Check sheet for the modelled part. Datum: model origin and axes. Units: mm. A direction names the side the tool comes from. Round coordinates to 2 decimals unless told otherwise and drop trailing zeros. Write each loop counter-clockwise with the first axis right and the second up, starting at its lowest first coordinate (ties: lowest second). Pieces come first, ordered by that corner, then holes. Notation, with made-up numbers: M 41.25,-24 L 50.25,-24 A25 cw 50.25,-4 Z; hole C 25.25,-15 d7. An arc over 180 degrees is marked long. Put each result on its own line as item: value.
```python
from build123d import *

# Parameters (mm, degrees)
F0_R     = 5
F0_R_2   = 3
F1_DEPTH = 20.162448287
F2_R     = 0.6272281394
F0_R_3   = 6
F3_DEPTH = 1.5


# Not quite as in the source:
# - a fillet or chamfer that OpenCascade refuses, or shapes differently, is made with other operations: its cross-section is extruded or revolved along the edge and cut away or added


with BuildPart() as f1:
    # F0 (on Front) → F1 (new body, symmetric)
    with BuildSketch(Plane.XZ):
        Circle(F0_R)
        Circle(F0_R_2, mode=Mode.SUBTRACT)
    extrude(amount=F1_DEPTH, both=True)

    # F2
    f2_edges = [f1.edges().sort_by_distance(p)[0] for p in [
        (-5, -20.162448, 0),
        (-5, 20.162448, 0),
    ]]
    fillet(f2_edges, radius=F2_R)

    # F0 (on Front) → F3 (join, symmetric)
    with BuildSketch(Plane.XZ):
        Circle(F0_R_3)
        Circle(F0_R, mode=Mode.SUBTRACT)
    extrude(amount=F3_DEPTH, both=True)

    # F4: fillet of radius 1.5182281224 on 2 edges, made by hand

    # F4_s1 → F4_t2 (revolve, cut)
    with BuildSketch(Plane.XY):
        with BuildLine():
            ThreePointArc((5, 1.5), (5.7251151811, 0.9442269358), (6, 0.072955416))
            Line((6, 0.072955416), (6, 1.5))
            Line((6, 1.5), (5, 1.5))
        make_face()
    revolve(axis=Axis((0, 1.5, 0), (0, -1, 0)), mode=Mode.SUBTRACT)

    # F4_s3 → F4_t4 (revolve, cut)
    with BuildSketch(Plane.XY):
        with BuildLine():
            ThreePointArc((6, -0.072955416), (5.7251151811, -0.9442269358), (5, -1.5))
            Line((5, -1.5), (6, -1.5))
            Line((6, -1.5), (6, -0.072955416))
        make_face()
    revolve(axis=Axis((0, -1.5, 0), (0, -1, 0)), mode=Mode.SUBTRACT)


solid = f1.part
```
1. Scan lines: probe 1 along Z at (x, y) = (0, -11); probe 2 along Z at (x, y) = (2.25, 1); probe 3 along Z at (x, y) = (-3.5, 18). Record each from-to range of solid material in increasing order.
Computed values:
probe 1: z = -5 to -3, 3 to 5
probe 2: z = -5.22 to -1.98, 1.98 to 5.22
probe 3: z = -3.57 to 3.57
2. Cross-section at C-C (y = -3.5). Enter the section's corners in (x, z).
Computed values:
outline: C 0,0 d10; hole C 0,0 d6
3. Access from +Z, -Z, +X, -X, +Y, -Y to the whole of each face (thin tool, end or side, straight path). Record for faces 4 (the cylindrical face through (-1.08, -10.64, -4.88)), 5 (the flat face through (-1, -20.162, -3)).
Computed values:
face 4: -Y
face 5: +Z, -Z, +X, -X, -Y
4. Depth check by flat-ended pin: pin 1 Ø1 at (x, y) = (-3.5, -10) entering from +Z; pin 2 Ø1.5 at (y, z) = (2.5, -0.5) entering from -X; pin 3 Ø1.5 at (y, z) = (-1.5, 0.5) entering from +X. Enter the tip coordinate at first touch or a pass-through.
Computed values:
pin 1: stops at z = 4
pin 2: stops at x = -5
pin 3: stops at x = 5.82
5. Cross-section at A-A (z = 0). Enter the section's corners in (x, y), then the cut area to 3 significant figures.
Computed values:
outline: M -6,-0.07 A1.52 ccw -5,-1.5 L -5,-19.54 A0.63 ccw -4.37,-20.16 L -3,-20.16 L -3,20.16 L -4.37,20.16 A0.63 ccw -5,19.54 L -5,1.5 A1.52 ccw -6,0.07 Z; M 3,-20.16 L 4.37,-20.16 A0.63 ccw 5,-19.54 L 5,-1.5 A1.52 ccw 6,-0.07 L 6,0.07 A1.52 ccw 5,1.5 L 5,19.54 A0.63 ccw 4.37,20.16 L 3,20.16 Z
area: 165 mm2
6. Release check for a two-part mould opening along X. For faces 1 (the cylindrical face through (-1.08, 10.39, -4.88)), 2 (the cylindrical face through (-3, 0, 0)), 3 (the flat face through (-1, 20.162, -3)) record: +X half, -X half, draft (parallel to the pull), parting line (faces both ways), or undercut.
Computed values:
face 1: parting line
face 2: undercut
face 3: draft
7. Cross-section at B-B (x = 0). Enter the section's corners in (y, z), then the cut area to 3 significant figures.
Computed values:
outline: M -20.16,-4.37 A0.63 ccw -19.54,-5 L -1.5,-5 A1.52 ccw -0.07,-6 L 0.07,-6 A1.52 ccw 1.5,-5 L 19.54,-5 A0.63 ccw 20.16,-4.37 L 20.16,-3 L -20.16,-3 Z; M -20.16,3 L 20.16,3 L 20.16,4.37 A0.63 ccw 19.54,5 L 1.5,5 A1.52 ccw 0.07,6 L -0.07,6 A1.52 ccw -1.5,5 L -19.54,5 A0.63 ccw -20.16,4.37 Z
area: 165 mm2
